Verification items for the finished model (mm, model axes). Give positions to 0.01 mm unless a question says otherwise; leave off trailing zeros. Loops run counter-clockwise (first coordinate to the right, second up) from the corner with the lowest first, then second, coordinate; pieces in that order, holes last. Notation, with made-up numbers: M 47.5,-25 L 98.5,-25 A15 ccw 98.5,-20 Z; hole C 57.25,-0.5 d1. An arc over 180 degrees is marked long. Use a Markdown table: item, result.
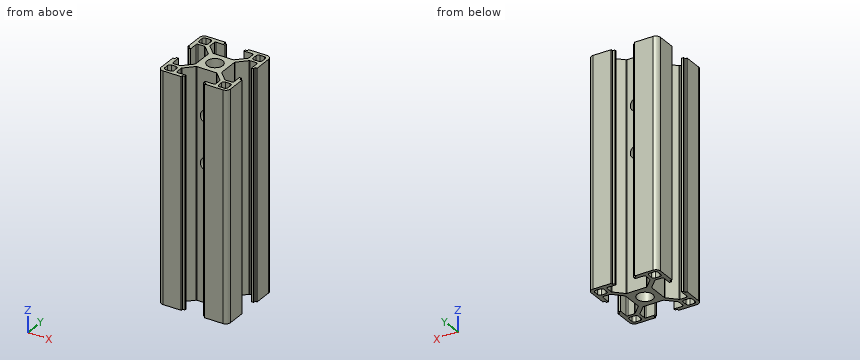
from build123d import *

# Parameters (mm, degrees)
SKETCH_1_W                       = 4
SKETCH_1_H                       = 4
EXTRUDE_1_DEPTH                  = 98.5
FILLET_1_R                       = 1
FILLET_2_R                       = 2
FILLET_3_R                       = 0.5
PATTERN_CIRCULAR_1_COUNT         = 4
FILLET_1_OF_PATTERN_CIRCULAR_1_R = 1
FILLET_2_OF_PATTERN_CIRCULAR_1_R = 2
FILLET_3_OF_PATTERN_CIRCULAR_1_R = 0.5
SKETCH_2_R                       = 3.4
CUT_EXTRUDE_1_DEPTH              = 99.5
SKETCH_3_R                       = 2.75
CUT_EXTRUDE_2_DEPTH              = 530


with BuildPart() as part:
    # 草图1 → 凸台-拉伸1 (new body)
    with BuildSketch(Plane.XY):
        Polygon((5.7, 0), (5.7, 4.427207794), (9.672792206, 8.4), (13.2, 8.4), (13.2, 4.1), (14.1, 4.1), (14.1, 5.1), (15, 5.1), (15, 15), (5.1, 15), (5.1, 14.1), (4.1, 14.1), (4.1, 13.2), (8.4, 13.2), (8.4, 9.672792206), (4.427207794, 5.7), (0, 5.7), (0, 0), align=None)
        with Locations((11.7, 11.7)):
            Rectangle(SKETCH_1_W, SKETCH_1_H, mode=Mode.SUBTRACT)
    extrude_1 = extrude(amount=EXTRUDE_1_DEPTH)

    # 圆角1
    fillet_1_edges = [part.edges().sort_by_distance(p)[0] for p in [
        (13.7, 9.7, 49.25),
        (13.7, 13.7, 49.25),
        (9.7, 13.7, 49.25),
        (9.7, 9.7, 49.25),
    ]]
    fillet(fillet_1_edges, radius=FILLET_1_R)

    # 圆角2
    fillet_2_edges = [part.edges().sort_by_distance(p)[0] for p in [
        (15, 15, 49.25),
    ]]
    fillet(fillet_2_edges, radius=FILLET_2_R)

    # 圆角3
    fillet_3_edges = [part.edges().sort_by_distance(p)[0] for p in [
        (4.427207794, 5.7, 49.25),
        (8.4, 9.672792206, 49.25),
        (8.4, 13.2, 49.25),
        (13.2, 8.4, 49.25),
        (9.672792206, 8.4, 49.25),
        (5.7, 4.427207794, 49.25),
    ]]
    fillet(fillet_3_edges, radius=FILLET_3_R)

    # 阵列(圆周)1: 凸台-拉伸1 ×4 about axis
    pattern_circular_1_axis = Axis((0, 0, 0), (0, 0, 1))
    for i in range(1, PATTERN_CIRCULAR_1_COUNT):
        add(extrude_1.rotate(pattern_circular_1_axis, i * 360 / PATTERN_CIRCULAR_1_COUNT))

    # 圆角1 of 阵列(圆周)1
    fillet_1_of_pattern_circular_1_edges = [part.edges().sort_by_distance(p)[0] for p in [
        (-9.7, 13.7, 49.25),
        (-13.7, 13.7, 49.25),
        (-13.7, 9.7, 49.25),
        (-9.7, 9.7, 49.25),
        (-13.7, -9.7, 49.25),
        (-13.7, -13.7, 49.25),
        (-9.7, -13.7, 49.25),
        (-9.7, -9.7, 49.25),
        (9.7, -13.7, 49.25),
        (13.7, -13.7, 49.25),
        (13.7, -9.7, 49.25),
        (9.7, -9.7, 49.25),
    ]]
    fillet(fillet_1_of_pattern_circular_1_edges, radius=FILLET_1_OF_PATTERN_CIRCULAR_1_R)

    # 圆角2 of 阵列(圆周)1
    fillet_2_of_pattern_circular_1_edges = [part.edges().sort_by_distance(p)[0] for p in [
        (-15, 15, 49.25),
        (-15, -15, 49.25),
        (15, -15, 49.25),
    ]]
    fillet(fillet_2_of_pattern_circular_1_edges, radius=FILLET_2_OF_PATTERN_CIRCULAR_1_R)

    # 圆角3 of 阵列(圆周)1
    fillet_3_of_pattern_circular_1_edges = [part.edges().sort_by_distance(p)[0] for p in [
        (-5.7, 4.427207794, 49.25),
        (-9.672792206, 8.4, 49.25),
        (-13.2, 8.4, 49.25),
        (-8.4, 13.2, 49.25),
        (-8.4, 9.672792206, 49.25),
        (-4.427207794, 5.7, 49.25),
        (-4.427207794, -5.7, 49.25),
        (-8.4, -9.672792206, 49.25),
        (-8.4, -13.2, 49.25),
        (-13.2, -8.4, 49.25),
        (-9.672792206, -8.4, 49.25),
        (-5.7, -4.427207794, 49.25),
        (5.7, -4.427207794, 49.25),
        (9.672792206, -8.4, 49.25),
        (13.2, -8.4, 49.25),
        (8.4, -13.2, 49.25),
        (8.4, -9.672792206, 49.25),
        (4.427207794, -5.7, 49.25),
    ]]
    fillet(fillet_3_of_pattern_circular_1_edges, radius=FILLET_3_OF_PATTERN_CIRCULAR_1_R)

    # 草图2 → 切除-拉伸1 (cut, through all)
    with BuildSketch(Plane.XY.offset(98.5)):
        Circle(SKETCH_2_R)
    extrude(amount=-CUT_EXTRUDE_1_DEPTH, mode=Mode.SUBTRACT)

    # 草图3 → 切除-拉伸2 (cut, symmetric)
    with BuildSketch(Plane(origin=(0, 0, 0), x_dir=(1, 0, 0), z_dir=(0, 1, 0))):
        with Locations((0, -58.5)):
            Circle(SKETCH_3_R)
        with Locations((0, -78.5)):
            Circle(SKETCH_3_R)
    extrude(amount=CUT_EXTRUDE_2_DEPTH, both=True, mode=Mode.SUBTRACT)


solid = part.part
(1) Cross-section at D-D on z = 58.5. State how many separate pieces and enclosed holes the cut face has, then the cut area to 3 significant figures.
Results below:
| item | result |
|---|---|
| separate pieces | 2 |
| enclosed holes | 4 |
| area | 263 mm^2 |
(2) Cross-section at A-A on y = 0. Record the cut outline in (x, z).
Results below:
| item | result |
|---|---|
| outline | M -5.7,0 L -3.4,0 L -3.4,98.5 L -5.7,98.5 Z; M 3.4,0 L 5.7,0 L 5.7,98.5 L 3.4,98.5 Z |
(3) Cross-section at C-C on y = -7. Record the cut outline in (x, z).
Results below:
| item | result |
|---|---|
| outline | M -15,0 L -13.2,0 L -13.2,98.5 L -15,98.5 Z; M -8.27,0 L -5.73,0 L -5.73,98.5 L -8.27,98.5 Z; M 5.73,0 L 8.27,0 L 8.27,98.5 L 5.73,98.5 Z; M 13.2,0 L 15,0 L 15,98.5 L 13.2,98.5 Z |
(4) Gauge pin test, flat ends, axial feed: P1, Ø6, axis at x = -10.5, y = -6, coming from the +Z side; P2, Ø3.5, axis at x = 0, z = 78.5, coming from the +Y side; P3, Ø0.7, axis at y = 14, z = 27.5, coming from the +X side; P4, Ø0.8, axis at x = 4.5, z = 59, coming from the +Y side. Record the tip position at first contact, or that the pin passes through.
Results below:
| item | result |
|---|---|
| P1 | z = 98.5 |
| P2 | through |
| P3 | x = 14.89 |
| P4 | y = 14.1 |
(5) Material ranges on line 1 (Z direction, x = 0, y = -4); line 2 (Y direction, x = 10.5, z = 42); line 3 (Y direction, x = 0, z = 62), recorded low to high.
Results below:
| item | result |
|---|---|
| line 1 | 0 to 55.75, 61.25 to 75.75, 81.25 to 98.5 |
| line 2 | -15 to -13.68, -9.72 to -8.4, 8.4 to 9.72, 13.68 to 15 |
| line 3 | -5.7 to -3.4, 3.4 to 5.7 |
(6) Cross-section at B-B on x = 0. Record the cut outline in (y, z).
Results below:
| item | result |
|---|---|
| outline | M -5.7,0 L -3.4,0 L -3.4,55.75 L -5.7,55.75 Z; M -5.7,61.25 L -3.4,61.25 L -3.4,75.75 L -5.7,75.75 Z; M -5.7,81.25 L -3.4,81.25 L -3.4,98.5 L -5.7,98.5 Z; M 3.4,0 L 5.7,0 L 5.7,55.75 L 3.4,55.75 Z; M 3.4,61.25 L 5.7,61.25 L 5.7,75.75 L 3.4,75.75 Z; M 3.4,81.25 L 5.7,81.25 L 5.7,98.5 L 3.4,98.5 Z |
